from build123d import *

# Parameters (mm, degrees)
BOSS_EXTRUDE1_DEPTH = 30
SKETCH2_R           = 2
CUT_EXTRUDE1_DEPTH  = 30


with BuildPart() as part:
    # Sketch1 → Boss-Extrude1 (new body)
    with BuildSketch(Plane(origin=(0, 0, 0), x_dir=(1, 0, 0), z_dir=(0, 1, 0))):
        with BuildLine():
            Line((10, 0), (20.95445115, 0))
            Line((20.95445115, 0), (21.95445115, 0))
            Line((21.95445115, 0), (21.95445115, 16))
            Line((21.95445115, 16), (20.95445115, 16))
            Line((20.95445115, 16), (20.95445115, 1))
            Line((20.95445115, 1), (10.95445115, 1))
            ThreePointArc((10.95445115, 1), (-0.500518406, 10.988606887), (-11, 0))
            Line((-11, 0), (-10, 0))
            ThreePointArc((-10, 0), (0, 10), (10, 0))
        make_face()
    extrude(amount=BOSS_EXTRUDE1_DEPTH)

    # Sketch2 → Cut-Extrude1 (cut)
    with BuildSketch(Plane(origin=(0, 0, -1), x_dir=(-1, 0, 0), z_dir=(0, 0, -1))):
        with Locations((-15.95445115, 25)):
            Circle(SKETCH2_R)
        with Locations((-15.95445115, 5)):
            Circle(SKETCH2_R)
    extrude(amount=-CUT_EXTRUDE1_DEPTH, mode=Mode.SUBTRACT)


solid = part.part
Here's how the part is built. I have some questions about the finished solid (model axes, mm). A direction names the side the tool comes from. Coordinates: 2 decimals unless noted, no trailing zeros. Order: outer loops, then holes, each group sorted by start corner. A loop starts at its lowest first (then second) coordinate and runs counter-clockwise, first axis right, second up. Notation, with made-up numbers: (14, 89) - (52, 89) arc R29 ccw to (52, 122) - close; hole circle Ø3 at (52.25, 52). An arc over 180 degrees is marked (long way). Use CSV: the item, a comma, the result in double quotes. Start each with the question number.
1. Suppose I cut it at A-A on y = 5. List the corners of the cut face in (x, z) for me.
2. Please list where these lines run through material, in increasing order: line 1 (X direction, y = 9.5, z = -7.5); line 2 (X direction, y = 9.25, z = -5.5); line 3 (Z direction, x = 19, y = 22.75). Write a range as from..to.
3. Suppose I cut it at C-C on z = -3. List the corners of the cut face in (x, y) for me, then the cut area to 3 significant figures.
4. I'm going to push flat-ended pins straight in: pin 1 (11 mm diameter, centred on x = 14.5, y = 15, fed in from -Z); pin 2 (2 mm diameter, centred on x = -7.5, y = 24, fed in from +Z); pin 3 (5 mm diameter, centred on y = 5.5, z = -8.5, fed in from -X). Where does each tip first touch, or does it pass through?
5. Suppose I cut it at B-B on y = 16.75. List the corners of the cut face in (x, z) for me.
6. Suppose I cut it at D-D on x = 15. List the corners of the cut face in (y, z) for me, then the cut area to 3 significant figures.
7. For faces 1 (the face through (16, 15, 0)), 2 (the face through (16, 15, -1)), which set-ups out of +Z, -Z, +X, -X, +Y, -Y let a thin tool reach every point of the face, with its end or its side?
8. If we mould it in two halves opening along X, with no side actions, what happens to faces 3 (the face through (9, 0, -6)), 4 (the face through (21.954, 15, -8)), 5 (the face through (0, 15, -10)), 6 (the face through (15.032, 23.226, -0.507))? For each: +X half, -X half, draft (parallel to the pull), parting line (faces both ways), or undercut.
Output:
1,outline,"(-11, 0) arc R11 ccw to (10.95, -1) - (13.95, -1) - (13.95, 0) - (10, 0) arc R10 cw to (-10, 0) - close; (17.95, -1) - (20.95, -1) - (20.95, -16) - (21.95, -16) - (21.95, 0) - (17.95, 0) - close"
2,line 1,"x = -8.05..-6.61, 6.61..8.05, 20.95..21.95"
2,line 2,"x = -9.53..-8.35, 8.35..9.53, 20.95..21.95"
2,line 3,"z = -1..0"
3,outline,"(-10.58, 0) - (-9.54, 0) - (-9.54, 30) - (-10.58, 30) - close; (9.54, 0) - (10.58, 0) - (10.58, 30) - (9.54, 30) - close; (20.95, 0) - (21.95, 0) - (21.95, 30) - (20.95, 30) - close"
3,area,"92.6 mm2"
4,pin 1,"stops at z = -6.32"
4,pin 2,"stops at z = -5.27"
4,pin 3,"stops at x = -9.22"
5,outline,"(-11, 0) arc R11 ccw to (10.95, -1) - (20.95, -1) - (20.95, -16) - (21.95, -16) - (21.95, 0) - (10, 0) arc R10 cw to (-10, 0) - close"
6,outline,"(0, -1) - (3.24, -1) - (3.24, 0) - (0, 0) - close; (6.76, -1) - (23.24, -1) - (23.24, 0) - (6.76, 0) - close; (26.76, -1) - (30, -1) - (30, 0) - (26.76, 0) - close"
6,area,"23.0 mm2"
7,face 1,"+Z, +X, -X, +Y, -Y"
7,face 2,"-Z, +Y, -Y"
8,face 3,"draft"
8,face 4,"+X half"
8,face 5,"undercut"
8,face 6,"undercut"
